Verification items for this drawing (mm, ordinates from the low corner). A direction names the side the tool comes from. Round coordinates to 2 decimals unless told otherwise and drop trailing zeros. Order: outer loops, then holes, each group sorted by start corner. A loop starts at its lowest first (then second) coordinate and runs counter-clockwise, first axis right, second up. Notation, with made-up numbers: (59.5, -13.5) -> (86.5, -13.5) arc R18 ccw to (86.5, 19.5) -> close; hole circle Ø9 at (-27, 35.5). An arc over 180 degrees is marked (long way). Answer in a Markdown table with one row per item.
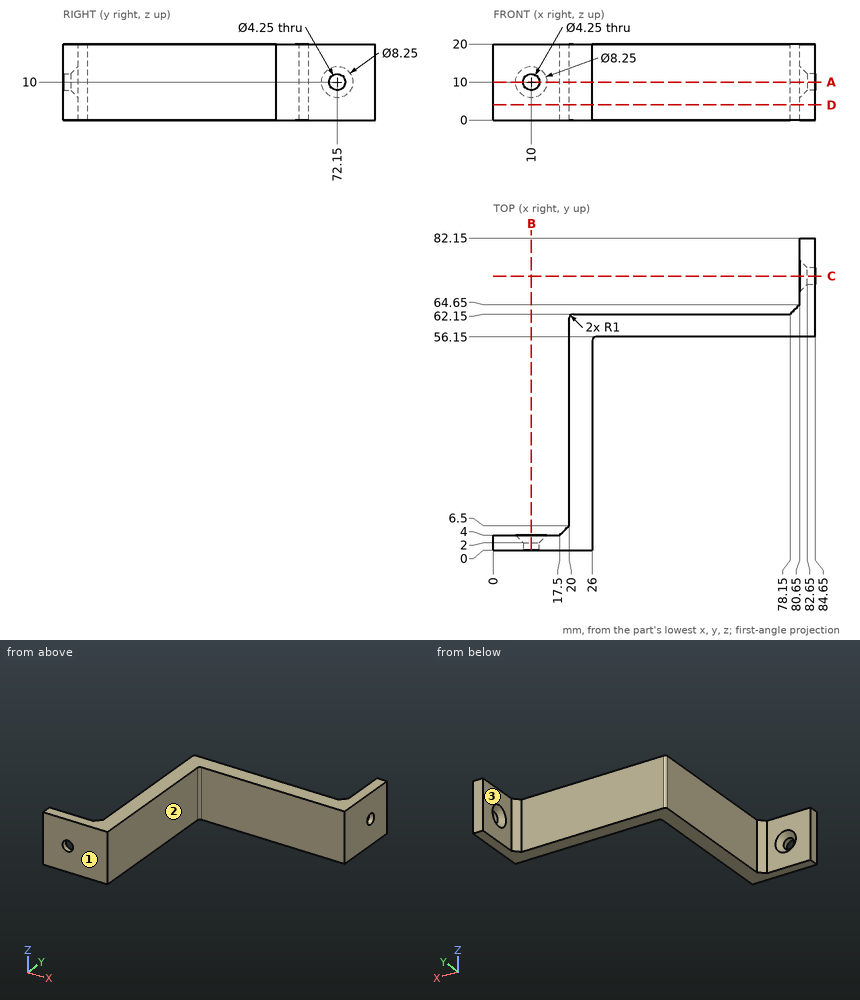
Item 1: Cross-section at A-A (z = 10). Record the boundary of the cut face in (x, y) (3 decimals).
Result sheet:
| item | result |
|---|---|
| outline | (0, 0) -> (7.875, 0) -> (7.875, 2) -> (5.875, 4) -> (0, 4) -> close; (12.125, 0) -> (26, 0) -> (26, 55.15) arc R1 cw to (27, 56.15) -> (84.65, 56.15) -> (84.65, 70.025) -> (82.65, 70.025) -> (80.65, 68.025) -> (80.65, 64.65) -> (78.15, 62.15) -> (21, 62.15) arc R1 ccw to (20, 61.15) -> (20, 6.5) -> (17.5, 4) -> (14.125, 4) -> (12.125, 2) -> close; (80.65, 76.275) -> (82.65, 74.275) -> (84.65, 74.275) -> (84.65, 82.15) -> (80.65, 82.15) -> close |
Item 2: Cross-section at B-B (x = 10). Record the boundary of the cut face in (y, z) (3 decimals).
Result sheet:
| item | result |
|---|---|
| outline | (0, 0) -> (4, 0) -> (4, 5.875) -> (2, 7.875) -> (0, 7.875) -> close; (0, 12.125) -> (2, 12.125) -> (4, 14.125) -> (4, 20) -> (0, 20) -> close |
Item 3: Scan lines: line 1 (Z direction, x = 10, y = 1.5) (3 decimals); line 2 (X direction, y = 65, z = 10); line 3 (Y direction, x = 44, z = 2). Record each from-to range of solid material in increasing order. Write a range as [from, to].
Result sheet:
| item | result |
|---|---|
| line 1 | z = [0, 7.875], [12.125, 20] |
| line 2 | x = [80.65, 84.65] |
| line 3 | y = [56.15, 62.15] |
Item 4: Set-up check for the marked faces 1, 2 and 3: record each of +Z, -Z, +X, -X, +Y, -Y from which the full face is reachable in a straight line by a thin tool's end or side.
Result sheet:
| item | result |
|---|---|
| face 1 | +Z, -Z, +X, -X, -Y |
| face 2 | +Z, -Z, +X, -Y |
| face 3 | +Z, -Z, -X, +Y |
Item 5: Cross-section at D-D (z = 4). Record the boundary of the cut face in (x, y).
Result sheet:
| item | result |
|---|---|
| outline | (0, 0) -> (26, 0) -> (26, 55.15) arc R1 cw to (27, 56.15) -> (84.65, 56.15) -> (84.65, 82.15) -> (80.65, 82.15) -> (80.65, 64.65) -> (78.15, 62.15) -> (21, 62.15) arc R1 ccw to (20, 61.15) -> (20, 6.5) -> (17.5, 4) -> (0, 4) -> close |
Item 6: Cross-section at C-C (y = 72.15). Record the boundary of the cut face in (x, z) (3 decimals), and give its area (3 significant figures).
Result sheet:
| item | result |
|---|---|
| outline | (80.65, 0) -> (84.65, 0) -> (84.65, 7.875) -> (82.65, 7.875) -> (80.65, 5.875) -> close; (80.65, 14.125) -> (82.65, 12.125) -> (84.65, 12.125) -> (84.65, 20) -> (80.65, 20) -> close |
| area | 59.0 mm^2 |
Item 7: Depth check by flat-ended pin: P1, Ø5, axis at x = 6, z = 14, coming from the +Y side; P2, Ø6, axis at y = 42.5, z = 8, coming from the -X side; P3, Ø6, axis at x = 58, z = 9, coming from the +Y side; P4, Ø2.5, axis at y = 72.15, z = 10, coming from the +X side. Enter the tip coordinate at first touch or a pass-through.
Result sheet:
| item | result |
|---|---|
| P1 | stops at y = 4 |
| P2 | stops at x = 20 |
| P3 | stops at y = 62.15 |
| P4 | passes through |
